For this review, take the finished solid that the model builds, in its own axes (mm). Round coordinates to 2 decimals unless told otherwise and drop trailing zeros. Loops run counter-clockwise (first coordinate to the right, second up) from the corner with the lowest first, then second, coordinate; pieces in that order, holes last.
1. Consider section B-B on z = 67. State the section outline as (x, y) points, then the cut area to 3 significant figures.
2. To check wall thickness, follow line 1 along X through (y, z) = (0.8, -16); line 2 along Z through (x, y) = (119.5, 0.3); line 3 along Z through (x, y) = (8.5, 0.75). State the ranges of each line that lie inside material, in increasing order.
3. Clearance check with flat-ended pins moving along their axes: pin 1 Ø0.5 at (y, z) = (0.5, 157.5) entering from -X; pin 2 Ø0.5 at (x, y) = (85.5, 0.5) entering from +Z; pin 3 Ø0.5 at (x, y) = (67.5, 0.5) entering from +Z. State where each tip first meets the part, or that it passes through.
from build123d import *

# Parameters (mm, degrees)
BOSS_EXTRUDE1_DEPTH = 1


with BuildPart() as part:
    # Sketch1 → Boss-Extrude1 (new body)
    with BuildSketch(Plane(origin=(0, 0, 0), x_dir=(1, 0, 0), z_dir=(0, 1, 0))):
        Polygon((0, 0), (2.5, 0), (2.5, 20), (7.5, 20), (7.5, 0), (42.5, 0), (42.5, 20), (47.5, 20), (47.5, 0), (82.5, 0), (82.5, 20), (87.5, 20), (87.5, 0), (100, 0), (100, -12.5), (120, -12.5), (120, -17.5), (100, -17.5), (100, -52.5), (120, -52.5), (120, -57.5), (100, -57.5), (100, -122.5), (120, -122.5), (120, -127.5), (100, -127.5), (100, -192.5), (120, -192.5), (120, -197.5), (100, -197.5), (100, -200), (150, -200), (150, 50), (0, 50), align=None)
    extrude(amount=BOSS_EXTRUDE1_DEPTH)


solid = part.part
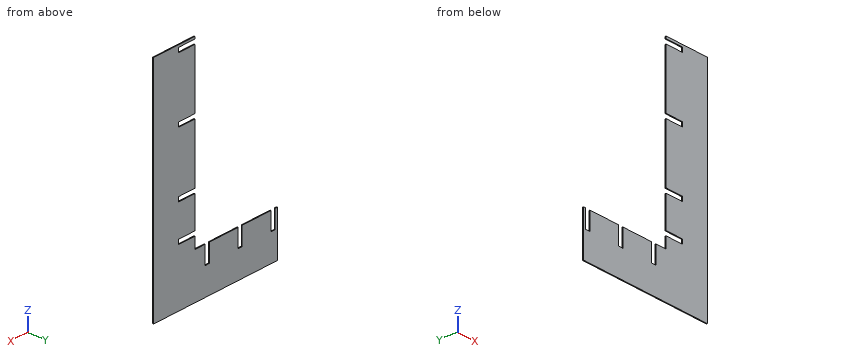
Resolved:
1. outline: (100, 0) - (150, 0) - (150, 1) - (100, 1) - close
1. area: 50.0 mm2
2. line 1: x = 0 to 2.5, 7.5 to 42.5, 47.5 to 82.5, 87.5 to 150
2. line 2: z = -50 to 12.5, 17.5 to 52.5, 57.5 to 122.5, 127.5 to 192.5, 197.5 to 200
2. line 3: z = -50 to 0
3. pin 1: stops at x = 100
3. pin 2: stops at z = -20
3. pin 3: stops at z = 0
